Verification items for the finished model (mm, model axes). A direction names the side the tool comes from. Give positions to 0.01 mm unless a question says otherwise; leave off trailing zeros. Loops run counter-clockwise (first coordinate to the right, second up) from the corner with the lowest first, then second, coordinate; pieces in that order, holes last. Notation, with made-up numbers: (-1.75, -8) - (30.25, -8) arc R31 cw to (30.25, 20) - close; hole circle Ø9 at (1, -0.5). An arc over 180 degrees is marked (long way). One line per item, written item: value. Start each with the question number.
1. Sectioned sample at C-C (z = -1). Record the cut outline in (x, y).
2. Access from +Z, -Z, +X, -X, +Y, -Y to the whole of each face (thin tool, end or side, straight path). Record for faces 4 (the cylindrical face through (-1.38, -0.62, -6.2)), 5 (the cylindrical face through (8.64, 29.96, 0.08)).
3. Scan lines: L1, parallel to Y at x = 8.05, z = 0; L2, parallel to Z at x = 0.5, y = 16. Record each from-to range of solid material in increasing order. Write a range as [from, to].
4. Sectioned sample at B-B (x = 8.25). Record the cut outline in (y, z), plus the area to 3 significant figures.
5. Gauge pin test, flat ends, axial feed: pin 1 (10 mm diameter, centred on y = -29.5, z = -2, fed in from -X); pin 2 (6 mm diameter, centred on x = 8.5, y = 16, fed in from -Z); pin 3 (2 mm diameter, centred on y = -22.5, z = 3, fed in from -X); pin 4 (3 mm diameter, centred on y = -31.75, z = 0, fed in from +X). Record the tip position at first contact, or that the pin passes through.
6. Mould release check, pull along Y, two halves, no side actions. Record for faces 1 (the flat face through (5, -44.45, -5)), 2 (the cylindrical face through (8.64, -33.54, 0.08)), 3 (the flat face through (5, 44.45, -5)): pulls with the +Y half, pulls with the -Y half, needs draft (parallel to the pull), parting line crosses it, or undercut.
from build123d import *

# Parameters (mm, degrees)
F0_W     = 22.225
F0_H     = 22.225
F1_DEPTH = 44.45
F2_R     = 1.7907
F3_DEPTH = 10.16
F4_R     = 1.7907
F5_DEPTH = 10.16
F7_DEPTH = 88.9
F8_R     = 6.35
F9_DEPTH = 88.9


with BuildPart() as f1:
    # F0 (on Front) → F1 (new body, symmetric)
    with BuildSketch(Plane.XZ):
        Rectangle(F0_W, F0_H)
    extrude(amount=F1_DEPTH, both=True)

    # F2 (on face) → F3 (cut)
    with BuildSketch(Plane.YZ.offset(11.1125)):
        with Locations((31.75, 0)):
            Circle(F2_R)
    extrude(amount=-F3_DEPTH, mode=Mode.SUBTRACT)

    # F4 (on face) → F5 (cut)
    with BuildSketch(Plane.YZ.offset(11.1125)):
        with Locations((-31.75, 0)):
            Circle(F4_R)
    extrude(amount=-F5_DEPTH, mode=Mode.SUBTRACT)

    # F6 (on face) → F7 (cut)
    with BuildSketch(Plane.XZ.offset(44.45)):
        with BuildLine():
            ThreePointArc((-11.1125, -4.55e-08), (-7.857724122, 7.8577240898), (0, 11.1125))
            Line((0, 11.1125), (-9.5319095999, 11.1125))
            Line((-9.5319095999, 11.1125), (-11.1125, 11.1125))
            Line((-11.1125, 11.1125), (-11.1125, -4.55e-08))
        make_face()
        with BuildLine():
            ThreePointArc((0, 11.1125), (7.8577241059, 7.8577241059), (11.1125, 0))
            Line((11.1125, 0), (11.1125, 11.1125))
            Line((11.1125, 11.1125), (0, 11.1125))
        make_face()
        with BuildLine():
            Line((11.1125, -11.1125), (11.1125, 0))
            ThreePointArc((11.1125, 0), (7.8577241059, -7.8577241059), (0, -11.1125))
            Line((0, -11.1125), (11.1125, -11.1125))
        make_face()
        with BuildLine():
            Line((-11.1125, -11.1125), (0, -11.1125))
            ThreePointArc((0, -11.1125), (-7.8577240898, -7.857724122), (-11.1125, -4.55e-08))
            Line((-11.1125, -4.55e-08), (-11.1125, -11.1125))
        make_face()
    extrude(amount=-F7_DEPTH, mode=Mode.SUBTRACT)

    # F8 (on face) → F9 (cut)
    with BuildSketch(Plane.XZ.offset(44.45)):
        Circle(F8_R)
    extrude(amount=-F9_DEPTH, mode=Mode.SUBTRACT)


solid = f1.part
Results are:
1. outline: (-11.07, -44.45) - (-6.27, -44.45) - (-6.27, 44.45) - (-11.07, 44.45) - close; (6.27, -44.45) - (11.07, -44.45) - (11.07, -33.24) - (6.27, -33.24) - close; (6.27, -30.26) - (11.07, -30.26) - (11.07, 30.26) - (6.27, 30.26) - close; (6.27, 33.24) - (11.07, 33.24) - (11.07, 44.45) - (6.27, 44.45) - close
2. face 4: +Y, -Y
2. face 5: +X
3. L1: y = [-44.45, -33.54], [-29.96, 29.96], [33.54, 44.45]
3. L2: z = [-11.1, -6.33], [6.33, 11.1]
4. outline: (-44.45, -7.44) - (44.45, -7.44) - (44.45, 7.44) - (-44.45, 7.44) - close; hole circle Ø3.58 at (-31.75, 0); hole circle Ø3.58 at (31.75, 0)
4. area: 1,300 mm^2
5. pin 1: stops at x = -11.11
5. pin 2: stops at z = -9.66
5. pin 3: stops at x = -10.93
5. pin 4: stops at x = -6.17
6. face 1: pulls with the -Y half
6. face 2: undercut
6. face 3: pulls with the +Y half
